```python
from build123d import *

# Parameters (mm, degrees)
SKETCH1_R               = 75.946
BOSS_EXTRUDE1_DEPTH     = 10.16
CUT_EXTRUDE4_DEPTH      = 11.16
SKETCH6_R               = 3.183478234
SKETCH6_R_2             = 3.2
SKETCH6_R_3             = 3.175
CUT_EXTRUDE5_DEPTH      = 1
CUT_EXTRUDE5_DEPTH_BACK = 11.16
SKETCH7_R               = 74.295
BOSS_EXTRUDE2_DEPTH     = 1.27
SKETCH8_R               = 3.183478234
SKETCH8_R_2             = 3.2
SKETCH8_R_3             = 3.175
CUT_EXTRUDE6_DEPTH      = 12.43
CUT_EXTRUDE7_DEPTH      = 12.43


with BuildPart() as part:
    # Sketch1 → Boss-Extrude1 (new body)
    with BuildSketch(Plane(origin=(0, 0, 0), x_dir=(1, 0, 0), z_dir=(0, 1, 0))):
        Circle(SKETCH1_R)
    extrude(amount=BOSS_EXTRUDE1_DEPTH)

    # Sketch5 → Cut-Extrude4 (cut, through all)
    with BuildSketch(Plane(origin=(0, 10.16, 0), x_dir=(1, 0, 0), z_dir=(0, 1, 0))):
        Polygon((0, 69.657309978), (-60.325, 34.828654989), (-60.325, -34.828654989), (0, -69.657309978), (60.325, -34.828654989), (60.325, 34.828654989), align=None)
    extrude(amount=-CUT_EXTRUDE4_DEPTH, mode=Mode.SUBTRACT)

    # Sketch6 → Cut-Extrude5 (cut, two sides)
    with BuildSketch(Plane(origin=(0, 10.16, 0), x_dir=(1, 0, 0), z_dir=(0, 1, 0))) as cut_extrude5_sk:
        with Locations((-67.945, 0)):
            Circle(SKETCH6_R)
        with Locations((-33.779572603, 58.808854795)):
            Circle(SKETCH6_R_2)
        with Locations((-33.953308147, -58.808854795)):
            Circle(SKETCH6_R_3)
        with Locations((33.953308147, -58.808854795)):
            Circle(SKETCH6_R_3)
        with Locations((67.945, 0)):
            Circle(SKETCH6_R)
        with Locations((33.779572603, 58.808854795)):
            Circle(SKETCH6_R_2)
    extrude(amount=CUT_EXTRUDE5_DEPTH, mode=Mode.SUBTRACT)
    extrude(cut_extrude5_sk.sketch, amount=-CUT_EXTRUDE5_DEPTH_BACK, mode=Mode.SUBTRACT)

    # Sketch7 → Boss-Extrude2 (add)
    with BuildSketch(Plane(origin=(0, 10.16, 0), x_dir=(1, 0, 0), z_dir=(0, 1, 0))):
        Circle(SKETCH7_R)
    extrude(amount=BOSS_EXTRUDE2_DEPTH)

    # Sketch8 → Cut-Extrude6 (cut, through all)
    with BuildSketch(Plane(origin=(0, 11.43, 0), x_dir=(1, 0, 0), z_dir=(0, 1, 0))):
        with Locations((-67.402457705, 0.180847432)):
            Circle(SKETCH8_R)
        with Locations((-44.45, 50.8)):
            Circle(SKETCH8_R_2)
        with Locations((-44.45, -50.8)):
            Circle(SKETCH8_R_3)
        with Locations((44.45, -50.8)):
            Circle(SKETCH8_R_3)
        with Locations((68.487542295, 0.180847432)):
            Circle(SKETCH8_R)
        with Locations((44.45, 50.8)):
            Circle(SKETCH8_R_2)
    extrude(amount=-CUT_EXTRUDE6_DEPTH, mode=Mode.SUBTRACT)

    # Sketch9 → Cut-Extrude7 (cut, through all)
    with BuildSketch(Plane(origin=(0, 11.43, 0), x_dir=(1, 0, 0), z_dir=(0, 1, 0))):
        Polygon((-0.180847432, 70.019004841), (-60.505847432, 35.190349852), (-60.505847432, -34.466960125), (-0.180847432, -69.295615114), (60.144152568, -34.466960125), (60.144152568, 35.190349852), align=None)
    extrude(amount=-CUT_EXTRUDE7_DEPTH, mode=Mode.SUBTRACT)


solid = part.part
```
The listing builds one solid part. Answer for the finished solid, in the listing's coordinates (mm). A direction names the side the tool comes from. Give positions to 0.01 mm unless a question says otherwise; leave off trailing zeros. Order: outer loops, then holes, each group sorted by start corner. A loop starts at its lowest first (then second) coordinate and runs counter-clockwise, first axis right, second up. Notation, with made-up numbers: (-5.5, 42) -> (33.5, 42) arc R19 ccw to (33.5, 53) -> close; hole circle Ø8 at (-37, -10.75). An arc over 180 degrees is marked (long way). Answer as CSV lines item,"result". Start each with the question number.
Q1. A cutting plane is placed at A-A (z = 17). Determine the outline of the cut face in (x, y) (3 decimals).
Q2. A cutting plane is placed at D-D (y = 7). Count the separate pieces of the cut face and the enclosed holes in it, then the cut area to 3 significant figures.
Q3. Given pin 1 (5 mm diameter, centred on x = 44.45, z = 50.8, fed in from +Y); pin 2 (1 mm diameter, centred on y = 4, z = -42, fed in from -X); pin 3 (7 mm diameter, centred on x = -35, z = 60, fed in from -Y); pin 4 (2 mm diameter, centred on y = 4.5, z = -54.5, fed in from +X), each flat-ended and moving along its own axis, determine where each tip first touches the part or whether it passes through.
Q4. A cutting plane is placed at C-C (z = 50.8). Determine the outline of the cut face in (x, y) (1 decimal), then the cut area to 3 significant figures.
Q5. A cutting plane is placed at B-B (x = -44.45). Determine the outline of the cut face in (y, z) (3 decimals), then the cut area to 3 significant figures.
Q6. Find the intervals of material crossed by L1, parallel to X at y = 5, z = 0 (3 decimals); L2, parallel to Z at x = -44.45, y = 3.5 (3 decimals); L3, parallel to X at y = 6.75, z = -50.8, in increasing order.
Q7. Determine the mould class of faces 1 (the flat face through (34, 10.16, 59)), 2 (the cylindrical face through (64.902, 5.151, 0.936)), 3 (the flat face through (33.4, 0, -51)) for opening direction Z: pulls with the +Z half, pulls with the -Z half, needs draft (parallel to the pull), parting line crosses it, or undercut.
Q8. Which of the six approach directions +Z, -Z, +X, -X, +Y, -Y give full straight-line access (tool end or side, diameter ignored) to faces 4 (the cylindrical face through (-34.473, 5.151, -55.685)), 5 (the flat face through (30.404, 5.795, -52.361))?
Results found:
1,outline,"(-74.019, 0) -> (-60.506, 0) -> (-60.506, 11.43) -> (-72.324, 11.43) -> (-72.324, 10.16) -> (-74.019, 10.16) -> close; (60.144, 10.16) -> (60.325, 10.16) -> (60.325, 0) -> (74.019, 0) -> (74.019, 10.16) -> (72.324, 10.16) -> (72.324, 11.43) -> (60.144, 11.43) -> close"
2,separate pieces,"1"
2,enclosed holes,"11"
2,area,"5,130 mm2"
3,pin 1,"through"
3,pin 2,"x = -63.6"
3,pin 3,"y = 0"
3,pin 4,"x = 53.9"
4,outline,"(-56.5, 0) -> (-47.6, 0) -> (-47.6, 11.4) -> (-54.2, 11.4) -> (-54.2, 10.2) -> (-56.5, 10.2) -> close; (-41.3, 0) -> (-32.7, 0) -> (-32.7, 10.2) -> (-32.2, 10.2) -> (-32.2, 11.4) -> (-41.3, 11.4) -> close; (31.9, 10.2) -> (32.7, 10.2) -> (32.7, 0) -> (41.3, 0) -> (41.3, 11.4) -> (31.9, 11.4) -> close; (47.6, 0) -> (56.5, 0) -> (56.5, 10.2) -> (54.2, 10.2) -> (54.2, 11.4) -> (47.6, 11.4) -> close"
4,area,"395 mm2"
5,outline,"(0, -61.579) -> (10.16, -61.579) -> (10.16, -59.531) -> (11.43, -59.531) -> (11.43, -54) -> (0, -54) -> close; (0, -47.6) -> (11.43, -47.6) -> (11.43, -44.46) -> (0, -44.46) -> close; (0, 43.994) -> (10.16, 43.994) -> (10.16, 43.737) -> (11.43, 43.737) -> (11.43, 47.625) -> (0, 47.625) -> close; (0, 53.975) -> (11.43, 53.975) -> (11.43, 59.531) -> (10.16, 59.531) -> (10.16, 61.579) -> (0, 61.579) -> close"
5,area,"246 mm2"
6,L1,"-75.946 to -71.128, -64.224 to -60.506, 60.325 to 64.762, 71.666 to 75.946"
6,L2,"-61.579 to -54, -47.6 to -44.46, 43.994 to 47.625, 53.975 to 61.579"
6,L3,"-56.45 to -47.65, -41.25 to -33.47, 33.11 to 41.25, 47.65 to 56.45"
7,face 1,"undercut"
7,face 2,"undercut"
7,face 3,"needs draft"
8,face 4,"-Y"
8,face 5,"+Y, -Y"
